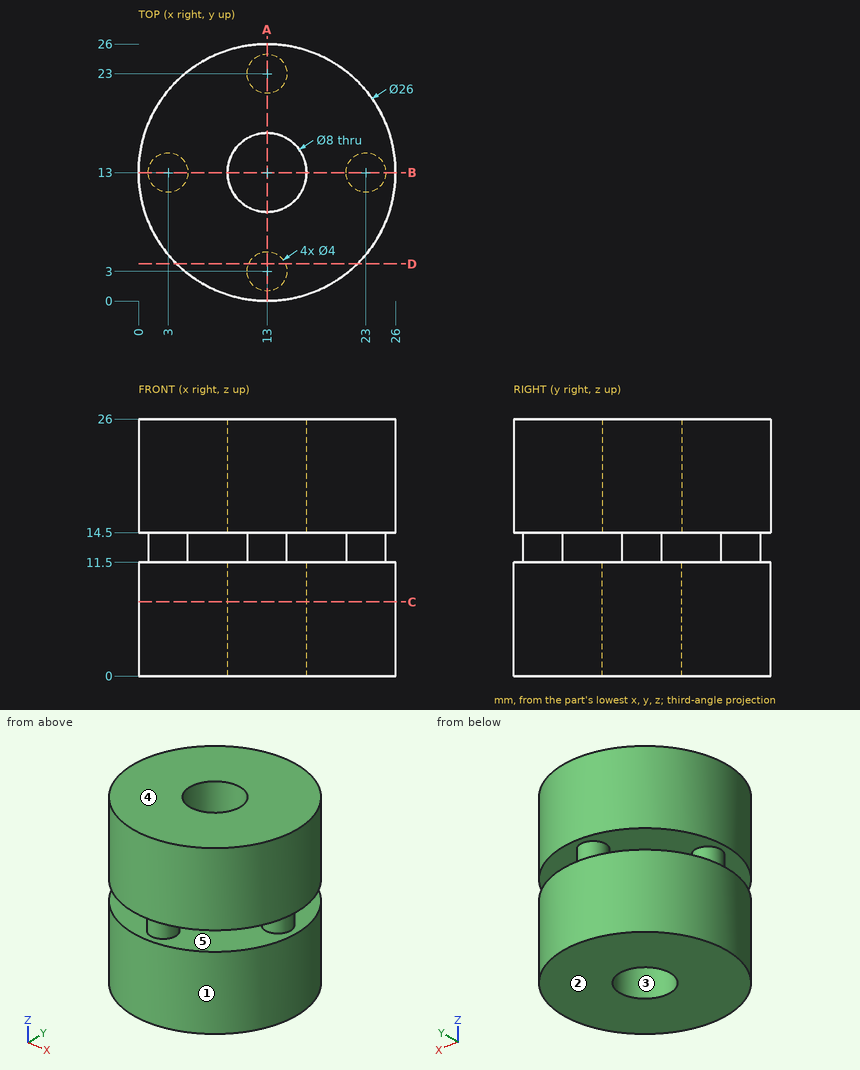
Check sheet for the drawn part. Datum: minimum x, y, z corner. Units: mm. A direction names the side the tool comes from. Round coordinates to 2 decimals unless told otherwise and drop trailing zeros. Loops run counter-clockwise (first coordinate to the right, second up) from the corner with the lowest first, then second, coordinate; pieces in that order, holes last. Notation, with made-up numbers: (76, 78.25) - (85, 78.25) arc R16 ccw to (85, 92.25) - close; hole circle Ø4 at (65.5, 5.5). An arc over 180 degrees is marked (long way). Write item = value, one per line. Start each with the question number.
1. Thickness scan on line 1 (Z direction, x = 11.5, y = 6.75); line 2 (Y direction, x = 13, z = 4); line 3 (X direction, y = 11.75, z = 21.5). Record the ranges inside material, lowest first.
2. Section check D-D on y = 3.75. Enter the section's corners in (x, z).
3. Set-up check for the marked faces 4 and 5: record each of +Z, -Z, +X, -X, +Y, -Y from which the full face is reachable in a straight line by a thin tool's end or side.
4. Depth check by flat-ended pin: pin 1 (10 mm diameter, centred on x = 10.5, y = 14, fed in from +Z); pin 2 (10 mm diameter, centred on x = 20.5, z = 7.5, fed in from -Y); pin 3 (1.5 mm diameter, centred on y = 6, z = 4.5, fed in from -X); pin 4 (3 mm diameter, centred on x = 11, z = 9, fed in from -Y). Enter the tip coordinate at first touch or a pass-through.
5. Section check C-C on z = 7.5. Enter the section's corners in (x, y), then the cut area to 3 significant figures.
6. Mould release check, pull along X, two halves, no side actions. Record for the marked faces 1, 2 and 3: released by +X, released by -X, zero draft, split by the parting line, or undercut.
7. Section check A-A on x = 13. Enter the section's corners in (y, z).
Working result:
q1.line_1 = 0 to 11.5, 14.5 to 26
q1.line_2 = 0 to 9, 17 to 26
q1.line_3 = 0.06 to 9.2, 16.8 to 25.94
q2.outline = (3.87, 0) - (22.13, 0) - (22.13, 11.5) - (14.85, 11.5) - (14.85, 14.5) - (22.13, 14.5) - (22.13, 26) - (3.87, 26) - (3.87, 14.5) - (11.15, 14.5) - (11.15, 11.5) - (3.87, 11.5) - close
q3.face_4 = +Z, +X, -X, +Y, -Y
q3.face_5 = none
q4.pin_1 = 26
q4.pin_2 = 0.24
q4.pin_3 = 1.6
q4.pin_4 = 0.01
q5.outline = circle Ø26 at (13, 13); hole circle Ø8 at (13, 13)
q5.area = 481 mm^2
q6.face_1 = split by the parting line
q6.face_2 = zero draft
q6.face_3 = undercut
q7.outline = (0, 0) - (9, 0) - (9, 11.5) - (5, 11.5) - (5, 14.5) - (9, 14.5) - (9, 26) - (0, 26) - (0, 14.5) - (1, 14.5) - (1, 11.5) - (0, 11.5) - close; (17, 0) - (26, 0) - (26, 11.5) - (25, 11.5) - (25, 14.5) - (26, 14.5) - (26, 26) - (17, 26) - (17, 14.5) - (21, 14.5) - (21, 11.5) - (17, 11.5) - close
